Input: dimensioned drawing with shaded views. Units: mm. Origin: part minimum x, y, z. A direction names the side the tool comes from. Round coordinates to 2 decimals unless told otherwise and drop trailing zeros. Write each loop counter-clockwise with the first axis right and the second up, starting at its lowest first coordinate (ties: lowest second). Pieces come first, ordered by that corner, then holes. Notation, with made-up numbers: (23.5, 79.25) - (28.5, 79.25) arc R28 ccw to (28.5, 107.25) - close; hole circle Ø4 at (68.5, 11). An arc over 180 degrees is marked (long way). Use one line per item in the form item = value.
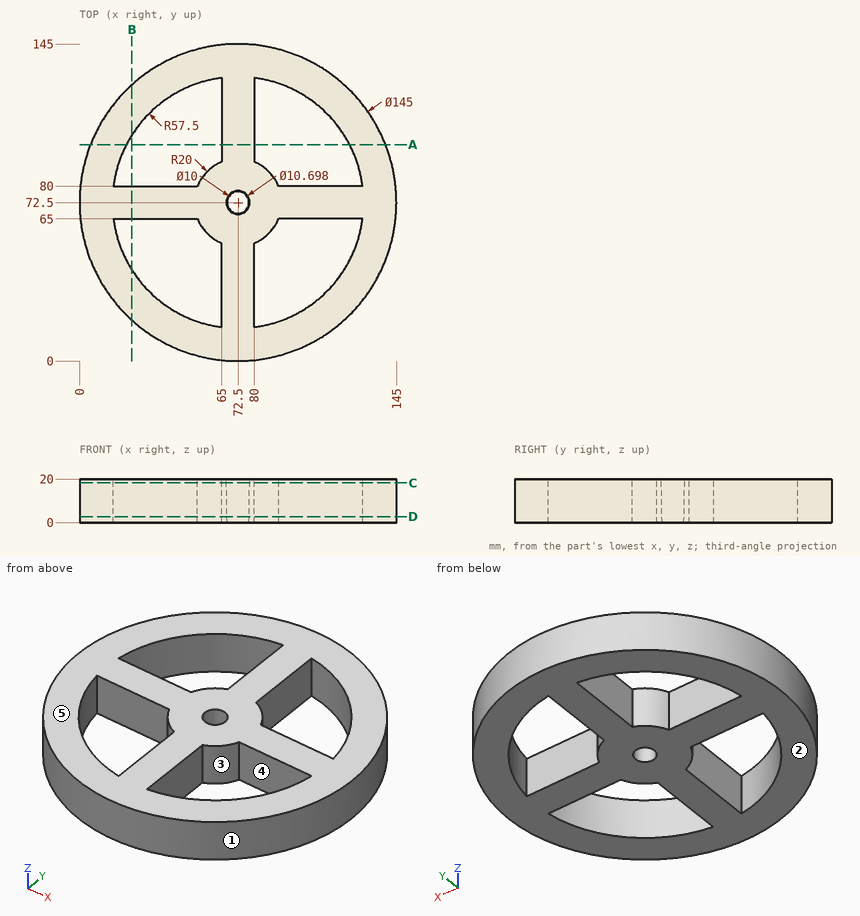
(1) First-contact query: pin 1 Ø4 at (x, z) = (124.5, 4.5) entering from -Y; pin 2 Ø6 at (y, z) = (116.5, 6) entering from +X; pin 3 Ø10 at (x, z) = (26.5, 12.5) entering from -Y; pin 4 Ø8 at (y, z) = (74.5, 9) entering from +X. Flat tips, straight axial feed; report the tip coordinate or a pass-through.
Derived:
pin_1 = 20
pin_2 = 132.29
pin_3 = 12.71
pin_4 = 145
(2) Access query for the marked faces 4 and 5. Directions: +Z, -Z, +X, -X, +Y, -Y. A direction counts if a zero-diameter tool reaches every point of the face in a straight line with its end or side. Return the directions, or none.
Derived:
face_4 = +Z, -Z
face_5 = +Z, +X, -X, +Y, -Y
(3) Draft query along Y for the marked faces 1, 2 and 3. Return one class per face: released by +Y, released by -Y, zero draft, split by the parting line, or undercut.
Derived:
face_1 = split by the parting line
face_2 = zero draft
face_3 = undercut
(4) Cut plane D-D on z = 2.75. Output: boundary loops of the cut face in (x, y).
Derived:
outline = circle Ø145 at (72.5, 72.5); hole (15.49, 65) arc R57.5 ccw to (65, 15.49) - (65, 53.96) arc R20 cw to (53.96, 65) - close; hole (15.49, 80) - (53.96, 80) arc R20 cw to (65, 91.04) - (65, 129.51) arc R57.5 ccw to start; hole circle Ø10.1 at (72.5, 72.5); hole (80, 15.49) arc R57.5 ccw to (129.51, 65) - (91.04, 65) arc R20 cw to (80, 53.96) - close; hole (80, 91.04) arc R20 cw to (91.04, 80) - (129.51, 80) arc R57.5 ccw to (80, 129.51) - close
(5) Cut plane B-B on x = 24. Output: boundary loops of the cut face in (y, z), then the cut area to 3 significant figures.
Derived:
outline = (18.61, 0) - (41.61, 0) - (41.61, 20) - (18.61, 20) - close; (65, 0) - (80, 0) - (80, 20) - (65, 20) - close; (103.39, 0) - (126.39, 0) - (126.39, 20) - (103.39, 20) - close
area = 1,220 mm^2
(6) Material intervals for L1, parallel to X at y = 81, z = 6.5; L2, parallel to Y at x = 117, z = 18.75 (1 decimal); L3, parallel to X at y = 59.5, z = 10.25 (1 decimal), sorted ascending.
Derived:
L1 = 0.5 to 15.63, 54.4 to 90.6, 129.37 to 144.5
L2 = 15.3 to 36.1, 65 to 80, 108.9 to 129.7
L3 = 1.2 to 16.5, 57.3 to 87.7, 128.5 to 143.8
(7) Cut plane A-A on y = 99. Output: boundary loops of the cut face in (x, z), then the cut area to 3 significant figures.
Derived:
outline = (5.02, 0) - (21.47, 0) - (21.47, 20) - (5.02, 20) - close; (65, 0) - (80, 0) - (80, 20) - (65, 20) - close; (123.53, 0) - (139.98, 0) - (139.98, 20) - (123.53, 20) - close
area = 958 mm^2
(8) Cut plane C-C on z = 18.25. Output: boundary loops of the cut face in (x, y), then the cut area to 3 significant figures.
Derived:
outline = circle Ø145 at (72.5, 72.5); hole (15.49, 65) arc R57.5 ccw to (65, 15.49) - (65, 53.96) arc R20 cw to (53.96, 65) - close; hole (15.49, 80) - (53.96, 80) arc R20 cw to (65, 91.04) - (65, 129.51) arc R57.5 ccw to start; hole circle Ø10.64 at (72.5, 72.5); hole (80, 15.49) arc R57.5 ccw to (129.51, 65) - (91.04, 65) arc R20 cw to (80, 53.96) - close; hole (80, 91.04) arc R20 cw to (91.04, 80) - (129.51, 80) arc R57.5 ccw to (80, 129.51) - close
area = 9,560 mm^2
